Read the model definition and answer for the solid it produces. Units are mm, in the model's axes. Face numbers are marked on the shaded views. Coordinates: 2 decimals unless noted, no trailing zeros. Write each loop counter-clockwise with the first axis right and the second up, starting at its lowest first coordinate (ties: lowest second). Pieces come first, ordered by that corner, then holes. Notation, with made-up numbers: (53, -20.5) -> (92, -20.5) arc R13 ccw to (92, -0.5) -> close; hole circle Ø10 at (34.25, -24). An arc over 180 degrees is marked (long way). Use CSV: the item, a comma, the result in double quotes.
from build123d import *

# Parameters (mm, degrees)
SKETCH1_W           = 45
SKETCH1_H           = 25
BOSS_EXTRUDE1_DEPTH = 70
SKETCH2_R           = 6
CUT_EXTRUDE1_DEPTH  = 70
SKETCH3_R           = 10
CUT_EXTRUDE2_DEPTH  = 2
SKETCH4_R           = 10
CUT_EXTRUDE3_DEPTH  = 2
SKETCH5_R           = 2.5
CUT_EXTRUDE4_DEPTH  = 15
SKETCH6_R           = 2.5
CUT_EXTRUDE5_DEPTH  = 15
SKETCH7_R           = 2.5
CUT_EXTRUDE6_DEPTH  = 36
SKETCH8_R           = 2.5
CUT_EXTRUDE7_DEPTH  = 38
SKETCH9_W           = 45
SKETCH9_H           = 25
BOSS_EXTRUDE2_DEPTH = 16
SKETCH10_W          = 45
SKETCH10_H          = 25
BOSS_EXTRUDE3_DEPTH = 16
SKETCH11_R          = 2.5
BOSS_EXTRUDE4_DEPTH = 25
SKETCH12_R          = 2.5
BOSS_EXTRUDE5_DEPTH = 27
SKETCH13_R          = 2.5
CUT_EXTRUDE8_DEPTH  = 14


with BuildPart() as part:
    # Sketch1 → Boss-Extrude1 (new body)
    with BuildSketch(Plane(origin=(0, 0, 0), x_dir=(1, 0, 0), z_dir=(0, 1, 0))):
        Rectangle(SKETCH1_W, SKETCH1_H)
    extrude(amount=BOSS_EXTRUDE1_DEPTH)

    # Sketch2 → Cut-Extrude1 (cut)
    with BuildSketch(Plane(origin=(22.5, 0, 0), x_dir=(0, 0, -1), z_dir=(1, 0, 0))):
        with Locations((0, 52.5)):
            Circle(SKETCH2_R)
        with Locations((0, 17.5)):
            Circle(SKETCH2_R)
    extrude(amount=-CUT_EXTRUDE1_DEPTH, mode=Mode.SUBTRACT)

    # Sketch3 → Cut-Extrude2 (cut)
    with BuildSketch(Plane(origin=(22.5, 0, 0), x_dir=(0, 0, -1), z_dir=(1, 0, 0))):
        with Locations((0, 17.5)):
            Circle(SKETCH3_R)
        with Locations((0, 52.5)):
            Circle(SKETCH3_R)
    extrude(amount=-CUT_EXTRUDE2_DEPTH, mode=Mode.SUBTRACT)

    # Sketch4 → Cut-Extrude3 (cut)
    with BuildSketch(Plane.ZY.offset(22.5)):
        with Locations((0, 52.5)):
            Circle(SKETCH4_R)
        with Locations((0, 17.5)):
            Circle(SKETCH4_R)
    extrude(amount=-CUT_EXTRUDE3_DEPTH, mode=Mode.SUBTRACT)

    # Sketch5 → Cut-Extrude4 (cut)
    with BuildSketch(Plane(origin=(22.5, 0, 0), x_dir=(0, 0, -1), z_dir=(1, 0, 0))):
        with Locations((7.5, 6)):
            Circle(SKETCH5_R)
        with Locations((-7.5, 6)):
            Circle(SKETCH5_R)
        with Locations((7.5, 64)):
            Circle(SKETCH5_R)
        with Locations((-7.5, 64)):
            Circle(SKETCH5_R)
    extrude(amount=-CUT_EXTRUDE4_DEPTH, mode=Mode.SUBTRACT)

    # Sketch6 → Cut-Extrude5 (cut)
    with BuildSketch(Plane(origin=(22.5, 0, 0), x_dir=(0, 0, -1), z_dir=(1, 0, 0))):
        with Locations((0, 35)):
            Circle(SKETCH6_R)
    extrude(amount=-CUT_EXTRUDE5_DEPTH, mode=Mode.SUBTRACT)

    # Sketch7 → Cut-Extrude6 (cut)
    with BuildSketch(Plane.XY.offset(12.5)):
        with Locations((-15.5, 52.5)):
            Circle(SKETCH7_R)
        with Locations((-15.5, 17.5)):
            Circle(SKETCH7_R)
    extrude(amount=-CUT_EXTRUDE6_DEPTH, mode=Mode.SUBTRACT)

    # Sketch8 → Cut-Extrude7 (cut)
    with BuildSketch(Plane.XY.offset(12.5)):
        with Locations((-15.5, 64)):
            Circle(SKETCH8_R)
        with Locations((-15.5, 6)):
            Circle(SKETCH8_R)
    extrude(amount=-CUT_EXTRUDE7_DEPTH, mode=Mode.SUBTRACT)

    # Sketch9 → Boss-Extrude2 (add)
    with BuildSketch(Plane(origin=(0, 70, 0), x_dir=(1, 0, 0), z_dir=(0, 1, 0))):
        Rectangle(SKETCH9_W, SKETCH9_H)
    extrude(amount=BOSS_EXTRUDE2_DEPTH)

    # Sketch10 → Boss-Extrude3 (add)
    with BuildSketch(Plane.XZ):
        Rectangle(SKETCH10_W, SKETCH10_H)
    extrude(amount=BOSS_EXTRUDE3_DEPTH)

    # Sketch11 → Boss-Extrude4 (add)
    with BuildSketch(Plane(origin=(0, 0, -12.5), x_dir=(-1, 0, 0), z_dir=(0, 0, -1))):
        with Locations((15.5, 64)):
            Circle(SKETCH11_R)
        with Locations((15.5, 6)):
            Circle(SKETCH11_R)
    extrude(amount=-BOSS_EXTRUDE4_DEPTH)

    # Sketch12 → Boss-Extrude5 (add)
    with BuildSketch(Plane(origin=(22.5, 0, 0), x_dir=(0, 0, -1), z_dir=(1, 0, 0))):
        with Locations((-7.5, 64)):
            Circle(SKETCH12_R)
        with Locations((7.5, 64)):
            Circle(SKETCH12_R)
        with Locations((-7.5, 6)):
            Circle(SKETCH12_R)
        with Locations((7.5, 6)):
            Circle(SKETCH12_R)
    extrude(amount=-BOSS_EXTRUDE5_DEPTH)

    # Sketch13 → Cut-Extrude8 (cut)
    with BuildSketch(Plane(origin=(0, 86, 0), x_dir=(1, 0, 0), z_dir=(0, 1, 0))):
        with Locations((18, 7.5)):
            Circle(SKETCH13_R)
        with Locations((-18, -7.5)):
            Circle(SKETCH13_R)
    extrude(amount=-CUT_EXTRUDE8_DEPTH, mode=Mode.SUBTRACT)


solid = part.part
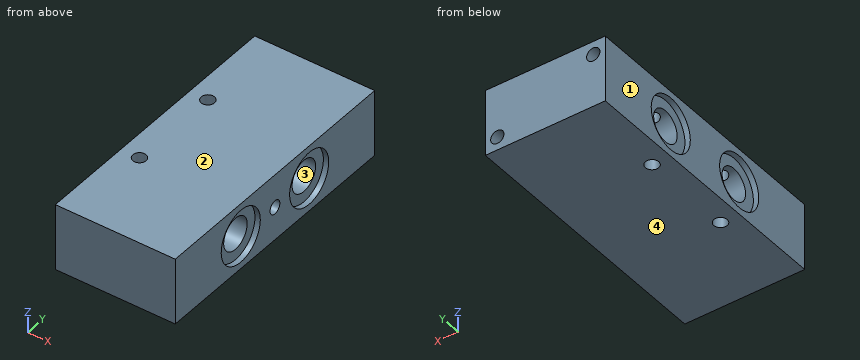
1. Each of these flat-tipped pins is pushed along its axis until it touches: pin 1 Ø4 at (x, z) = (-18, 7.5) entering from +Y; pin 2 Ø4.5 at (x, y) = (-15.5, 52.5) entering from -Z; pin 3 Ø10 at (y, z) = (48.5, 1) entering from +X; pin 4 Ø6 at (y, z) = (48, 4.5) entering from -X. Where does it stop, or does it pass through?
Solutions:
pin 1,"stops at y = 72"
pin 2,"passes through"
pin 3,"stops at x = 20.5"
pin 4,"stops at x = -20.5"
2. A cutting plane is placed at A-A (y = 52.5). Give the vertices of the cut face in (x, z), and give its area (3 significant figures).
Solutions:
outline,"(-22.5, -12.5) -> (-18, -12.5) -> (-18, -6) -> (-20.5, -6) -> (-20.5, -10) -> (-22.5, -10) -> close; (-22.5, 10) -> (-20.5, 10) -> (-20.5, 6) -> (-18, 6) -> (-18, 12.5) -> (-22.5, 12.5) -> close; (-13, -12.5) -> (22.5, -12.5) -> (22.5, -10) -> (20.5, -10) -> (20.5, -6) -> (-13, -6) -> close; (-13, 6) -> (20.5, 6) -> (20.5, 10) -> (22.5, 10) -> (22.5, 12.5) -> (-13, 12.5) -> close"
area,"488 mm^2"
3. Find the intervals of material crossed by line 1 along Y through (x, z) = (-21.55, 0); line 2 along Y through (x, z) = (-15.5, 8.25); line 3 along Z through (x, y) = (-21, 52), in increasing order.
Solutions:
line 1,"y = -16 to 7.5, 27.5 to 42.5, 62.5 to 86"
line 2,"y = -16 to 15, 20 to 50, 55 to 86"
line 3,"z = -12.5 to -9.99, 9.99 to 12.5"
4. For a pull along Z with two mould halves and no side action, classify the marked faces 1, 2, 3 and 4 as pulls with the +Z half, pulls with the -Z half, needs draft (parallel to the pull), parting line crosses it, or undercut.
Solutions:
face 1,"needs draft"
face 2,"pulls with the +Z half"
face 3,"undercut"
face 4,"pulls with the -Z half"
5. A cutting plane is placed at C-C (z = 4). Give the vertices of the cut face in (x, y).
Solutions:
outline,"(-22.5, -16) -> (22.5, -16) -> (22.5, 8.33) -> (20.5, 8.33) -> (20.5, 13.03) -> (-20.5, 13.03) -> (-20.5, 8.33) -> (-22.5, 8.33) -> close; (-22.5, 26.67) -> (-20.5, 26.67) -> (-20.5, 21.97) -> (20.5, 21.97) -> (20.5, 26.67) -> (22.5, 26.67) -> (22.5, 43.33) -> (20.5, 43.33) -> (20.5, 48.03) -> (-20.5, 48.03) -> (-20.5, 43.33) -> (-22.5, 43.33) -> close; (-22.5, 61.67) -> (-20.5, 61.67) -> (-20.5, 56.97) -> (20.5, 56.97) -> (20.5, 61.67) -> (22.5, 61.67) -> (22.5, 86) -> (-22.5, 86) -> close"
6. A cutting plane is placed at D-D (y = 79). Give the vertices of the cut face in (x, z).
Solutions:
outline,"(-22.5, -12.5) -> (22.5, -12.5) -> (22.5, 12.5) -> (-22.5, 12.5) -> close; hole circle Ø5 at (-18, 7.5); hole circle Ø5 at (18, -7.5)"
7. A cutting plane is placed at B-B (x = 12.5). Give the vertices of the cut face in (y, z).
Solutions:
outline,"(-16, -12.5) -> (86, -12.5) -> (86, 12.5) -> (-16, 12.5) -> close; hole circle Ø12 at (17.5, 0); hole circle Ø5 at (35, 0); hole circle Ø12 at (52.5, 0)"
